For this review, use the dimensioned drawing (mm, ordinates from the lowest corner) and the shaded views. Round coordinates to 2 decimals unless told otherwise and drop trailing zeros. Answer as CSV lines item,"result". Start each with the question number.
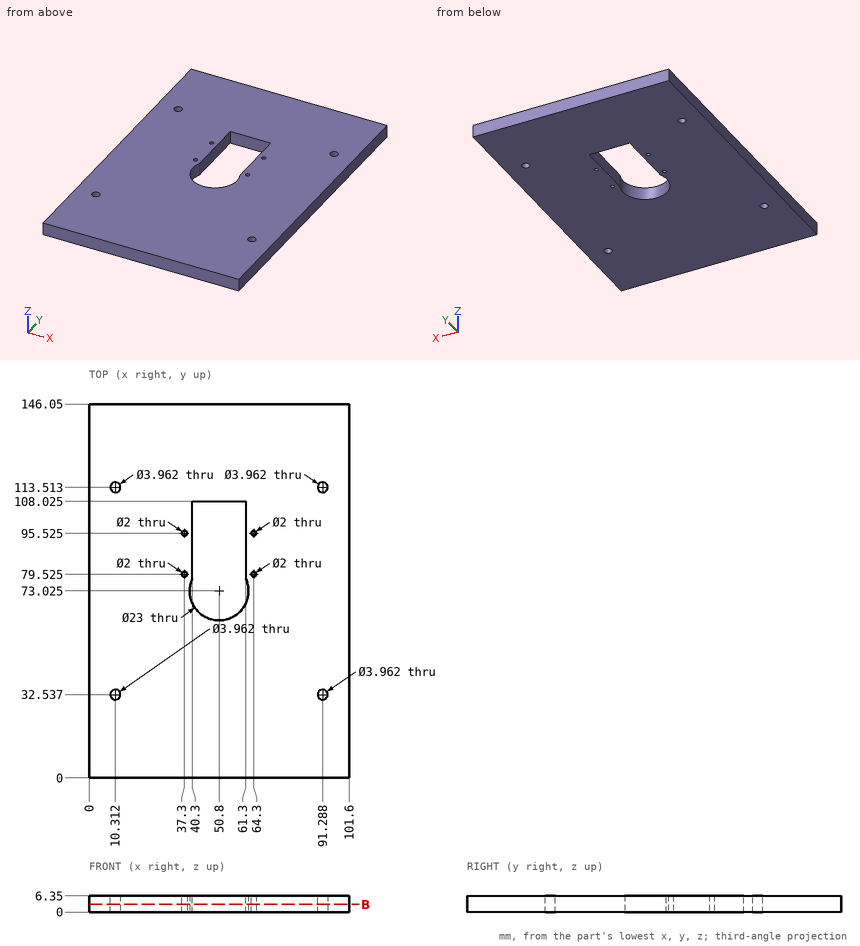
Item 1: Consider section B-B (z = 3). State how many separate pieces and enclosed holes the cut face has, and give its area (3 significant figures).
Item 2: Wall thickness on probe 1 along Y at (x, z) = (91, 3); probe 2 along X at (y, z) = (99.5, 1.5); probe 3 along X at (y, z) = (31, 1.5) (1 decimal): over which ranges is each line inside the solid? List them lowest first. Write a range as [from, to].
Item 3: For pin 1 (1.6 mm diameter, centred on x = 37.3, y = 95.525, fed in from -Z); pin 2 (2.5 mm diameter, centred on x = 64.3, y = 79.525, fed in from +Z), all flat-tipped, find the tip position at first contact; note any pin that passes through.
Reported:
1,separate pieces,"1"
1,enclosed holes,"9"
1,area,"13,800 mm²"
2,probe 1,"y = [0, 30.58], [34.5, 111.55], [115.47, 146.05]"
2,probe 2,"x = [0, 40.3], [61.3, 101.6]"
2,probe 3,"x = [0, 9.1], [11.6, 90], [92.5, 101.6]"
3,pin 1,"passes through"
3,pin 2,"stops at z = 6.35"
